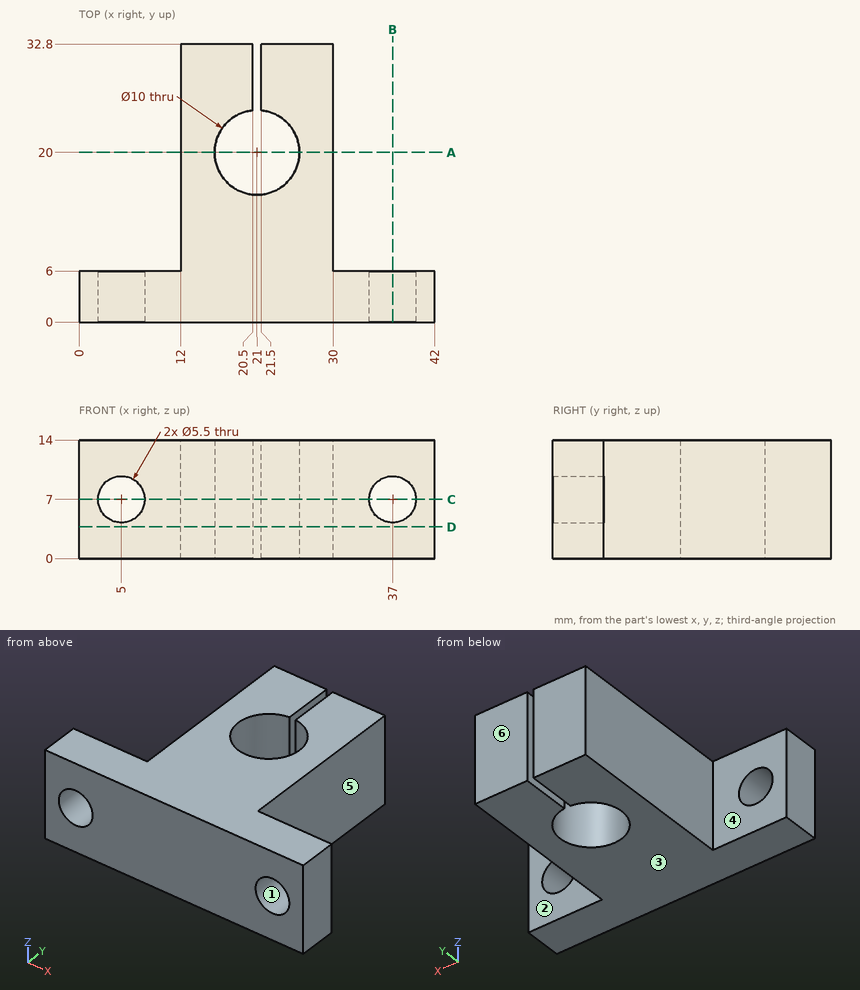
Input: dimensioned drawing with shaded views. Units: mm. Origin: part minimum x, y, z. A direction names the side the tool comes from. Give positions to 0.01 mm unless a question says otherwise; leave off trailing zeros. Write each loop counter-clockwise with the first axis right and the second up, starting at its lowest first coordinate (ties: lowest second). Pieces come first, ordered by that corner, then holes. Notation, with made-up numbers: (74, 83.25) -> (104, 83.25) arc R24 cw to (104, 93.25) -> close; hole circle Ø4 at (26, 2). An arc over 180 degrees is marked (long way). Return JSON: item names as keys, results as strings. Group by question number.
1. Section B-B, the plane x = 37. Output: boundary loops of the cut face in (y, z).
2. Section D-D, the plane z = 3.75. Output: boundary loops of the cut face in (x, y).
3. Access query for the marked faces 4, 5 and 6. Directions: +Z, -Z, +X, -X, +Y, -Y. A direction counts if a zero-diameter tool reaches every point of the face in a straight line with its end or side. Return the directions, or none.
4. Section A-A, the plane y = 20. Output: boundary loops of the cut face in (x, z), then the cut area to 3 significant figures.
5. Material intervals for line 1 (X direction, y = 2.2, z = 7); line 2 (X direction, y = 28, z = 8.75); line 3 (Z direction, x = 5, y = 4.65), sorted ascending. Write a range as from..to.
6. Mould query, pull axis Z, two halves, no side actions, for the marked faces 1, 2 and 3. Classes: +Z half, -Z half, draft (parallel to the pull), parting line (faces both ways), or undercut.
7. Section C-C, the plane z = 7. Output: boundary loops of the cut face in (x, y).
8. Pin query (flat end, axial travel): pin 1 Ø6.5 at (y, z) = (29, 10) entering from -X; pin 2 Ø6 at (x, z) = (8.5, 6.5) entering from +Y; pin 3 Ø4 at (y, z) = (24.5, 9) entering from +X. Return the tip coordinate at first contact, or that it passes through.
Determined:
{
 "1": {"outline": "(0, 0) -> (6, 0) -> (6, 4.25) -> (0, 4.25) -> close; (0, 9.75) -> (6, 9.75) -> (6, 14) -> (0, 14) -> close"},
 "2": {"outline": "(0, 0) -> (42, 0) -> (42, 6) -> (30, 6) -> (30, 32.8) -> (21.5, 32.8) -> (21.5, 24.97) arc R5 cw (long way) to (20.5, 24.97) -> (20.5, 32.8) -> (12, 32.8) -> (12, 6) -> (0, 6) -> close"},
 "3": {"face 4": "+Z, -Z, -X, +Y", "face 5": "+Z, -Z, +X, +Y", "face 6": "+Z, -Z, +X, -X, +Y"},
 "4": {"outline": "(12, 0) -> (16, 0) -> (16, 14) -> (12, 14) -> close; (26, 0) -> (30, 0) -> (30, 14) -> (26, 14) -> close", "area": "112 mm2"},
 "5": {"line 1": "x = 0..2.25, 7.75..34.25, 39.75..42", "line 2": "x = 12..20.5, 21.5..30", "line 3": "z = 0..4.25, 9.75..14"},
 "6": {"face 1": "undercut", "face 2": "draft", "face 3": "-Z half"},
 "7": {"outline": "(0, 0) -> (2.25, 0) -> (2.25, 6) -> (0, 6) -> close; (7.75, 0) -> (34.25, 0) -> (34.25, 6) -> (30, 6) -> (30, 32.8) -> (21.5, 32.8) -> (21.5, 24.97) arc R5 cw (long way) to (20.5, 24.97) -> (20.5, 32.8) -> (12, 32.8) -> (12, 6) -> (7.75, 6) -> close; (39.75, 0) -> (42, 0) -> (42, 6) -> (39.75, 6) -> close"},
 "8": {"pin 1": "stops at x = 12", "pin 2": "stops at y = 6", "pin 3": "stops at x = 30"}
}
